from build123d import *

# Parameters (mm, degrees)
BOSS_EXTRUDE1_DEPTH = 4
CUT_EXTRUDE1_DEPTH  = 4


with BuildPart() as part:
    # Sketch1 → Boss-Extrude1 (new body)
    with BuildSketch(Plane(origin=(0, 0, 0), x_dir=(1, 0, 0), z_dir=(0, 1, 0))):
        with BuildLine():
            Line((25, -20), (-25, -20))
            ThreePointArc((-25, -20), (-28.535533906, -18.535533906), (-30, -15))
            Line((-30, -15), (-30, 15))
            ThreePointArc((-30, 15), (-28.535533906, 18.535533906), (-25, 20))
            Line((-25, 20), (25, 20))
            ThreePointArc((25, 20), (28.535533906, 18.535533906), (30, 15))
            Line((30, 15), (30, -15))
            ThreePointArc((30, -15), (28.535533906, -18.535533906), (25, -20))
        make_face()
    extrude(amount=BOSS_EXTRUDE1_DEPTH)

    # Sketch2 → Cut-Extrude1 (cut)
    with BuildSketch(Plane(origin=(0, 4, 0), x_dir=(1, 0, 0), z_dir=(0, 1, 0))):
        with BuildLine():
            Line((-25, 17), (-20, 17))
            ThreePointArc((-20, 17), (-18, 15), (-20, 13))
            Line((-20, 13), (-25, 13))
            ThreePointArc((-25, 13), (-27, 15), (-25, 17))
        make_face()
        with BuildLine():
            Line((25, 17), (20, 17))
            ThreePointArc((20, 17), (18, 15), (20, 13))
            Line((20, 13), (25, 13))
            ThreePointArc((25, 13), (27, 15), (25, 17))
        make_face()
        with BuildLine():
            Line((25, -17), (20, -17))
            ThreePointArc((20, -17), (18, -15), (20, -13))
            Line((20, -13), (25, -13))
            ThreePointArc((25, -13), (27, -15), (25, -17))
        make_face()
        with BuildLine():
            Line((-25, -17), (-20, -17))
            ThreePointArc((-20, -17), (-18, -15), (-20, -13))
            Line((-20, -13), (-25, -13))
            ThreePointArc((-25, -13), (-27, -15), (-25, -17))
        make_face()
    extrude(amount=-CUT_EXTRUDE1_DEPTH, mode=Mode.SUBTRACT)


solid = part.part
Verification items for the finished model (mm, model axes). A direction names the side the tool comes from. Round coordinates to 2 decimals unless told otherwise and drop trailing zeros. Write each loop counter-clockwise with the first axis right and the second up, starting at its lowest first coordinate (ties: lowest second). Pieces come first, ordered by that corner, then holes.
(1) Access from +Z, -Z, +X, -X, +Y, -Y to the whole of each face (thin tool, end or side, straight path). Record for faces 4 (the cylindrical face through (-29, 2, -18)), 5 (the cylindrical face through (-27, 2, 15)).
Returned:
face 4: -Z, -X, +Y, -Y
face 5: +Y, -Y
(2) Section check A-A (x = 24). Enter the section's corners in (y, z).
Returned:
outline: (0, -20) - (4, -20) - (4, -17) - (0, -17) - close; (0, -13) - (4, -13) - (4, 13) - (0, 13) - close; (0, 17) - (4, 17) - (4, 20) - (0, 20) - close
(3) Mould release check, pull along Z, two halves, no side actions. Record for faces 1 (the flat face through (-30, 2, 0)), 2 (the flat face through (0, 2, 20)), 3 (the cylindrical face through (18, 2, -15)): pulls with the +Z half, pulls with the -Z half, needs draft (parallel to the pull), parting line crosses it, or undercut.
Returned:
face 1: needs draft
face 2: pulls with the +Z half
face 3: undercut
(4) Material ranges on line 1 (Z direction, x = 24, y = 0.8); line 2 (X direction, y = 0.85, z = -16.5); line 3 (Z direction, x = 26, y = 1.5), recorded low to high.
Returned:
line 1: z = -20 to -17, -13 to 13, 17 to 20
line 2: x = -29.77 to -26.32, -18.68 to 18.68, 26.32 to 29.77
line 3: z = -19.9 to -16.73, -13.27 to 13.27, 16.73 to 19.9
(5) Section check B-B (y = 2.6). Enter the section's corners in (x, z), plus the area to 3 significant figures.
Returned:
outline: (-30, -15) arc R5 ccw to (-25, -20) - (25, -20) arc R5 ccw to (30, -15) - (30, 15) arc R5 ccw to (25, 20) - (-25, 20) arc R5 ccw to (-30, 15) - close; hole (-25, -17) - (-20, -17) arc R2 ccw to (-20, -13) - (-25, -13) arc R2 ccw to start; hole (-25, 13) - (-20, 13) arc R2 ccw to (-20, 17) - (-25, 17) arc R2 ccw to start; hole (20, -17) - (25, -17) arc R2 ccw to (25, -13) - (20, -13) arc R2 ccw to start; hole (20, 13) - (25, 13) arc R2 ccw to (25, 17) - (20, 17) arc R2 ccw to start
area: 2,250 mm2
